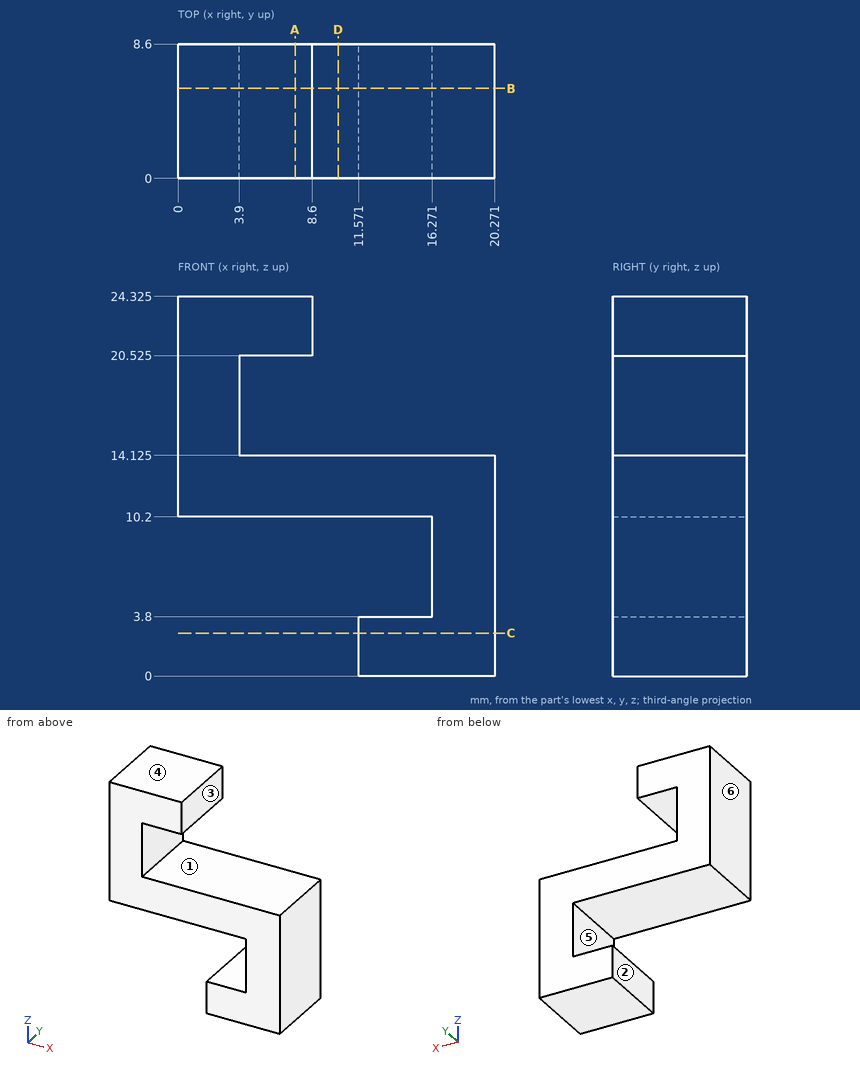
Here's the drawing with two shaded views (mm, measured from the low corner). I have some questions. A direction names the side the tool comes from. Round coordinates to 2 decimals unless told otherwise and drop trailing zeros. Loops run counter-clockwise (first coordinate to the right, second up) from the corner with the lowest first, then second, coordinate; pieces in that order, holes last.
Item 1: Suppose I cut it at B-B, the plane y = 5.75. Write out the boundary of the cut face in (x, z) (1 decimal).
Item 2: Suppose I cut it at A-A, the plane x = 7.5. Write out the boundary of the cut face in (y, z) (3 decimals).
Item 3: Suppose I cut it at D-D, the plane x = 10.25. Write out the boundary of the cut face in (y, z) (3 decimals).
Item 4: Will these pins go through, and if not, where does the flat tip stop? pin 1 Ø4 at (y, z) = (5.5, 21.5) entering from +X; pin 2 Ø5 at (x, y) = (14, 4) entering from +Z (3 decimals); pin 3 Ø1.5 at (y, z) = (3.5, 4.5) entering from -X.
Item 5: If we mould it in two halves opening along Z, with no side actions, what happens to the marked faces 4, 5 and 6? For each: +Z half, -Z half, draft (parallel to the pull), parting line (faces both ways), or undercut.
Item 6: Which directions (+Z, -Z, +X, -X, +Y, -Y) give clear straight access to the entire face, cutting with the end or side of a thin tool? Please do the marked faces 1, 2 and 3.
Item 7: Suppose I cut it at C-C, the plane z = 2.75. Write out the boundary of the cut face in (x, y), then the cut area to 3 significant figures.
Item 8: Please list where these lines run through material, in increasing order: L1, parallel to Z at x = 6.25, y = 4.25 (3 decimals); L2, parallel to Z at x = 13, y = 2 (3 decimals); L3, parallel to X at y = 0.75, z = 14.5.
Reported:
1. outline: (0, 10.2) - (16.3, 10.2) - (16.3, 3.8) - (11.6, 3.8) - (11.6, 0) - (20.3, 0) - (20.3, 14.1) - (3.9, 14.1) - (3.9, 20.5) - (8.6, 20.5) - (8.6, 24.3) - (0, 24.3) - close
2. outline: (0, 10.2) - (8.6, 10.2) - (8.6, 14.125) - (0, 14.125) - close; (0, 20.525) - (8.6, 20.525) - (8.6, 24.325) - (0, 24.325) - close
3. outline: (0, 10.2) - (8.6, 10.2) - (8.6, 14.125) - (0, 14.125) - close
4. pin 1: stops at x = 8.6
4. pin 2: stops at z = 14.125
4. pin 3: stops at x = 11.57
5. face 4: +Z half
5. face 5: undercut
5. face 6: draft
6. face 1: +X, +Y, -Y
6. face 2: -Z, -X, +Y, -Y
6. face 3: +Z, +X, +Y, -Y
7. outline: (11.57, 0) - (20.27, 0) - (20.27, 8.6) - (11.57, 8.6) - close
7. area: 74.8 mm2
8. L1: z = 10.2 to 14.125, 20.525 to 24.325
8. L2: z = 0 to 3.8, 10.2 to 14.125
8. L3: x = 0 to 3.9
